Autodesk Inventor part; units mm, degrees
ref_plane "YZ Plane" through (0, 0, 0) normal (1, 0, 0) x (0, 1, 0)
ref_plane "XZ Plane" through (0, 0, 0) normal (0, 1, 0) x (-1, 0, 0)
ref_plane "XY Plane" through (0, 0, 0) normal (0, 0, 1) x (1, 0, 0)
sketch "Sketch1" plane through (0, 0, 0) normal (0, 0, 1) x (1, 0, 0)
  line L0 (5.75, -21.6) -> (5.75, 21.6)
  line L1 (5.75, 21.6) -> (-5.75, 21.6)
  line L2 (-5.75, 21.6) -> (-5.75, -21.6)
  line L3 (-5.75, -21.6) -> (5.75, -21.6)
  circle A0 centre (-1.75, -18.4) radius 1.5
  circle A1 centre (-1.75, 17.6) radius 1.5
  circle A2 centre (-1.75, -0.4) radius 1.5
  line L4 (-12.75, -21.6) -> (-12.75, 21.6)
  line L5 (-12.75, 21.6) -> (-24.25, 21.6)
  line L6 (-24.25, 21.6) -> (-24.25, -21.6)
  line L7 (-24.25, -21.6) -> (-12.75, -21.6)
  circle A3 centre (-16.75, 17.6) radius 1.5
  circle A4 centre (-16.75, -0.4) radius 1.5
  circle A5 centre (-16.75, -18.4) radius 1.5
  line L8 (5.75, -21.6) -> (-24.25, -21.6)
  line L9 (-24.25, -21.6) -> (-24.25, 21.6)
  line L10 (-24.25, 21.6) -> (5.75, 21.6)
  line L11 (5.75, 21.6) -> (5.75, -21.6)
  point P0 (0, 0)
extrude "Extrusion1" add sketch "Sketch1" along normal blind 2
sketch "Sketch2" plane through (0, 0, 0) normal (0, 0, -1) x (-1, 0, 0)
  line L0 (-5.75, -21.6) -> (-5.75, 21.6)
  line L1 (24.25, -21.6) -> (-5.75, -21.6)
  line L2 (24.25, 21.6) -> (24.25, -21.6)
  line L3 (-5.75, 21.6) -> (24.25, 21.6)
  circle A0 centre (16.75, -18.4) radius 1.5
  circle A1 centre (16.75, -0.4) radius 1.5
  circle A2 centre (16.75, 17.6) radius 1.5
  circle A3 centre (1.75, -0.4) radius 1.5
  circle A4 centre (1.75, 17.6) radius 1.5
  circle A5 centre (1.75, -18.4) radius 1.5
  line L4 (5.2, 10.6) -> (5.2, -18.6)
  line L5 (-5.75, 10.6) -> (5.2, 10.6)
  line L6 (-5.75, -21.6) -> (-5.75, 21.6)
  line L7 (24.25, -18.6) -> (24.25, 10.6)
  line L8 (13.3, -18.6) -> (13.3, 10.6)
  line L9 (5.2, -18.6) -> (5.2, -21.6)
  line L10 (13.3, -21.6) -> (13.3, -18.6)
  line L11 (13.3, 10.6) -> (24.25, 10.6)
  line L12 (-5.75, 10.6) -> (5.2, 10.6)
  circle A6 centre (1.75, -0.4) radius 1.75
  circle A7 centre (1.75, 6.1) radius 1.5
  circle A8 centre (16.75, 6.1) radius 1.5
  circle A9 centre (16.75, -0.4) radius 1.75
  point P0 (0, 0)
  point P1 (18.2695, -1.2681)
extrude "Extrusion2" cut sketch "Sketch2" against normal blind 10 contours L0 L3 L2 L11 L8 L10 L1 L9 L4 L5 | A7 | A8
sketch "Sketch3" plane through (0, 0, 0) normal (0, 0, -1) x (-1, 0, 0)
  line L0 (5.2, -21.6) -> (-5.75, -21.6)
  line L1 (13.3, 10.6) -> (24.25, 10.6)
  line L2 (24.25, -9.4) -> (24.25, 8.7)
  line L3 (24.25, -18.6) -> (24.25, 10.6)
  line L4 (-5.75, -21.6) -> (-5.75, 10.6)
  line L5 (24.25, 10.6) -> (24.25, -21.6)
  line L6 (24.25, 10.6) -> (-5.75, 10.6)
  line L7 (-5.75, 10.6) -> (-5.75, -21.6)
  line L8 (-5.75, -21.6) -> (24.25, -21.6)
  line L9 (24.25, -21.6) -> (24.25, 10.6)
  line L10 (5.2, -21.6) -> (5.2, 10.6)
  line L11 (13.3, 10.6) -> (13.3, -21.6)
  point P0 (0, 0)
extrude "Extrusion3" add sketch "Sketch3" against normal blind 2 contours L10 L6 L11 L8
sketch "Sketch4" plane through (0, 0, 0) normal (0, 0, -1) x (-1, 0, 0)
  circle A0 centre (1.75, -18.4) radius 1.5
  circle A1 centre (1.75, -0.4) radius 1.5
  circle A2 centre (1.75, 6.1) radius 1.5
  line L0 (24.25, -21.6) -> (-5.75, -21.6)
  line L1 (24.25, 10.6) -> (24.25, -21.6)
  line L2 (24.25, 10.6) -> (-5.75, 10.6)
  line L3 (-5.75, -21.6) -> (-5.75, 10.6)
  circle A3 centre (16.75, 6.1) radius 1.5
  circle A4 centre (16.75, -18.4) radius 1.5
  circle A5 centre (16.75, -0.4) radius 1.5
  line L4 (-5.75, 10.6) -> (24.25, 10.6)
  line L5 (-5.75, -21.6) -> (-5.75, 10.6)
  line L6 (24.25, 10.6) -> (-5.75, 10.6)
  line L7 (-5.75, 10.6) -> (-5.75, 9.6)
  line L8 (-5.75, 9.6) -> (24.25, 9.6)
  line L9 (24.25, 9.6) -> (24.25, 10.6)
  point P0 (0, 0)
  dimension "d6" = 1
extrude "Extrusion4" cut sketch "Sketch4" against normal blind 2 contours L8 L3 L2 L1
properties part number "lead_3" material "Lead"
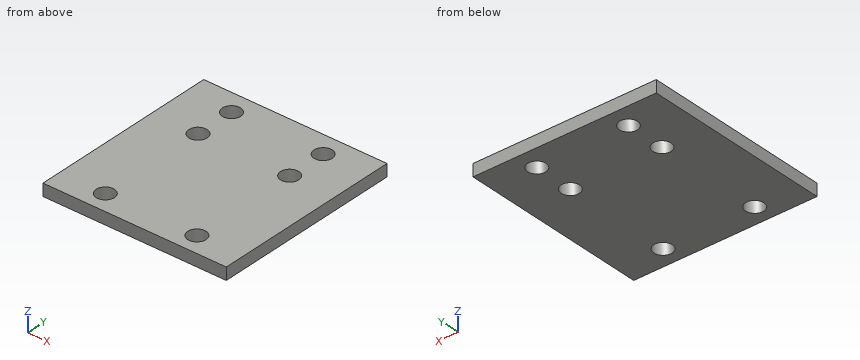
The model under review builds one solid part; all positions refer to its coordinate system, in mm. Give positions to 0.01 mm unless a question says otherwise; leave off trailing zeros. Loops run counter-clockwise (first coordinate to the right, second up) from the corner with the lowest first, then second, coordinate; pieces in that order, holes last. Notation, with made-up numbers: (12, 64.25) -> (54, 64.25) arc R27 cw to (54, 86.25) -> close; hole circle Ø6 at (77.5, 56.5). An arc over 180 degrees is marked (long way). Put each result on its own line as item: value. Start each with the question number.
1. We need section B-B on x = -1.75. State the section outline as (y, z) points, then the cut area to 3 significant figures.
2. We need section C-C on z = 0.3. State the section outline as (x, y) points.
3. Wall thickness on probe 1 along Y at (x, z) = (-16.75, 1.35); probe 2 along Y at (x, z) = (-3, 1.4): over which ranges is each line inside the solid? List them lowest first.
4. We need section A-A on y = -18.4. State the section outline as (x, z) points.
Determined:
1. outline: (-21.6, 0) -> (-19.9, 0) -> (-19.9, 2) -> (-21.6, 2) -> close; (-16.9, 0) -> (-1.9, 0) -> (-1.9, 2) -> (-16.9, 2) -> close; (1.1, 0) -> (4.6, 0) -> (4.6, 2) -> (1.1, 2) -> close; (7.6, 0) -> (9.6, 0) -> (9.6, 2) -> (7.6, 2) -> close
1. area: 44.4 mm^2
2. outline: (-24.25, -21.6) -> (5.75, -21.6) -> (5.75, 9.6) -> (-24.25, 9.6) -> close; hole circle Ø3 at (-16.75, -18.4); hole circle Ø3 at (-16.75, -0.4); hole circle Ø3 at (-16.75, 6.1); hole circle Ø3 at (-1.75, -18.4); hole circle Ø3 at (-1.75, -0.4); hole circle Ø3 at (-1.75, 6.1)
3. probe 1: -21.6 to -19.9, -16.9 to -1.9, 1.1 to 4.6, 7.6 to 9.6
3. probe 2: -21.6 to -19.23, -17.57 to -1.23, 0.43 to 5.27, 6.93 to 9.6
4. outline: (-24.25, 0) -> (-18.25, 0) -> (-18.25, 2) -> (-24.25, 2) -> close; (-15.25, 0) -> (-3.25, 0) -> (-3.25, 2) -> (-15.25, 2) -> close; (-0.25, 0) -> (5.75, 0) -> (5.75, 2) -> (-0.25, 2) -> close
